Build history of the part. All positions in model axes, mm. Round coordinates to 2 decimals unless told otherwise and drop trailing zeros. Loops run counter-clockwise (first coordinate to the right, second up) from the corner with the lowest first, then second, coordinate; pieces in that order, holes last. Notation, with made-up numbers: (7, 33.25) - (26, 33.25) arc R28 ccw to (26, 57.25) - close; hole circle Ø1 at (-5.5, -36). An arc over 180 degrees is marked (long way). One line per question, with ' | ' between items. Start each with the question number.
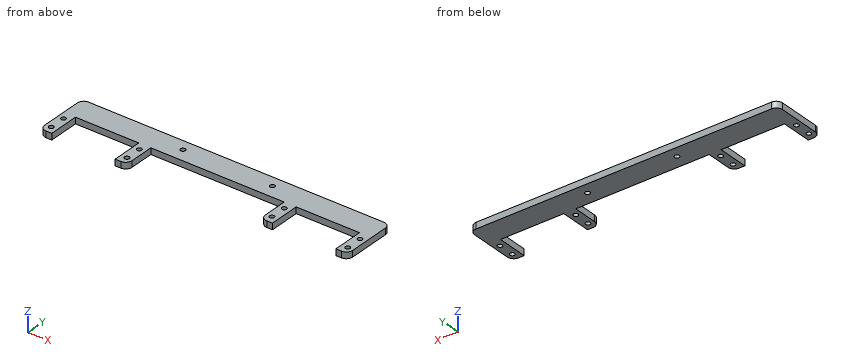
from build123d import *

# Parameters (mm, degrees)
BOSS_EXTRUDE2_DEPTH = 4
FILLET1_R           = 4
SKETCH6_R           = 1.5
CUT_EXTRUDE1_DEPTH  = 4
SKETCH3_R           = 1.5
CUT_EXTRUDE2_DEPTH  = 4


with BuildPart() as part:
    # Sketch2 → Boss-Extrude2 (new body)
    with BuildSketch(Plane.XY):
        Polygon((-67.081093968, -2.634474623), (-67.081093968, 16.923525377), (-26.695093968, 16.923525377), (-26.695093968, -2.634474623), (-19.075093968, -2.634474623), (-19.075093968, 32.365525377), (-67.081093968, 32.365525377), (-74.701093968, 32.365525377), (-159.701093968, 32.365525377), (-167.321093968, 32.365525377), (-215.327093968, 32.365525377), (-215.327093968, -2.634474623), (-207.707093968, -2.634474623), (-207.707093968, 16.923525377), (-167.321093968, 16.923525377), (-167.231910297, 16.736340115), (-167.321093968, 16.736752562), (-167.321093968, -2.634474623), (-159.701093968, -2.634474623), (-159.701093968, 16.923525377), (-74.701093968, 16.923525377), (-74.701093968, -2.634474623), align=None)
    extrude(amount=BOSS_EXTRUDE2_DEPTH)

    # Fillet1
    fillet1_edges = [part.edges().sort_by_distance(p)[0] for p in [
        (-19.075093968, 32.365525377, 2),
        (-19.075093968, -2.634474623, 2),
        (-74.701093968, -2.634474623, 2),
        (-159.701093968, -2.634474623, 2),
        (-215.327093968, -2.634474623, 2),
        (-215.327093968, 32.365525377, 2),
    ]]
    fillet(fillet1_edges, radius=FILLET1_R)

    # Sketch6 → Cut-Extrude1 (cut)
    with BuildSketch(Plane.XY.offset(4)):
        with Locations((-211.644093968, 12.224525377)):
            Circle(SKETCH6_R)
        with Locations((-163.384093968, 12.224525377)):
            Circle(SKETCH6_R)
        with Locations((-163.384093968, 2.064525377)):
            Circle(SKETCH6_R)
        with Locations((-211.644093968, 2.064525377)):
            Circle(SKETCH6_R)
        with Locations((-71.018093968, 12.224525377)):
            Circle(SKETCH6_R)
        with Locations((-22.758093968, 12.224525377)):
            Circle(SKETCH6_R)
        with Locations((-22.758093968, 2.064525377)):
            Circle(SKETCH6_R)
        with Locations((-71.018093968, 2.064525377)):
            Circle(SKETCH6_R)
    extrude(amount=-CUT_EXTRUDE1_DEPTH, mode=Mode.SUBTRACT)

    # Sketch3 → Cut-Extrude2 (cut)
    with BuildSketch(Plane.XY.offset(4)):
        with Locations((-145.701093968, 25.365525377)):
            Circle(SKETCH3_R)
        with Locations((-88.701093968, 25.365525377)):
            Circle(SKETCH3_R)
    extrude(amount=-CUT_EXTRUDE2_DEPTH, mode=Mode.SUBTRACT)


solid = part.part
1) Saw through at A-A on y = 8.5. Write the cut outline in (x, z), and give its area (3 significant figures).
2) Saw through at C-C on x = -53. Write the cut outline in (y, z).
3) Saw through at B-B on z = 1.8. State how many separate pieces and enclosed holes the cut face has, and give its area (3 significant figures).
4) Drop flat-ended pins along their axis: pin 1 (1.2 mm diameter, centred on x = -186.5, z = 1, fed in from -Y); pin 2 (1.8 mm diameter, centred on x = -71.02, y = 2.06, fed in from +Z). Give the stop position or say it passes through.
5) Wall check: line 1 (X direction, y = 8.5, z = 0.6); line 2 (X direction, y = 26, z = 1.5); line 3 (Y direction, x = -57, z = 1.9). Give the ranges that are in metal, low to high. Write a range as [from, to].
Answer key:
1) outline: (-215.33, 0) - (-207.71, 0) - (-207.71, 4) - (-215.33, 4) - close; (-167.32, 0) - (-159.7, 0) - (-159.7, 4) - (-167.32, 4) - close; (-74.7, 0) - (-67.08, 0) - (-67.08, 4) - (-74.7, 4) - close; (-26.7, 0) - (-19.08, 0) - (-19.08, 4) - (-26.7, 4) - close | area: 122 mm²
2) outline: (16.92, 0) - (32.37, 0) - (32.37, 4) - (16.92, 4) - close
3) separate pieces: 1 | enclosed holes: 10 | area: 3,540 mm²
4) pin 1: y = 16.92 | pin 2: through
5) line 1: [-215.33, -207.71], [-167.32, -159.7], [-74.7, -67.08], [-26.7, -19.08] | line 2: [-215.33, -147.06], [-144.34, -90.06], [-87.34, -19.08] | line 3: [16.92, 32.37]
